For this review, take the finished solid that the model builds, in its own axes (mm). Face numbers are marked on the shaded views. Coordinates: 2 decimals unless noted, no trailing zeros. Write each loop counter-clockwise with the first axis right and the second up, starting at its lowest first coordinate (ties: lowest second). Pieces come first, ordered by that corner, then holes.
```python
from build123d import *

# Parameters (mm, degrees)
CROQUIS1_W              = 44
CROQUIS1_H              = 35.7
CROQUIS1_R              = 14
SALIENTE_EXTRUIR1_DEPTH = 5.4


with BuildPart() as part:
    # Croquis1 → Saliente-Extruir1 (new body)
    with BuildSketch(Plane.XY):
        Rectangle(CROQUIS1_W, CROQUIS1_H)
        with Locations(Location((0, 0, 0), (0, 0, 180))):
            Circle(CROQUIS1_R, mode=Mode.SUBTRACT)
    extrude(amount=SALIENTE_EXTRUIR1_DEPTH)


solid = part.part
```
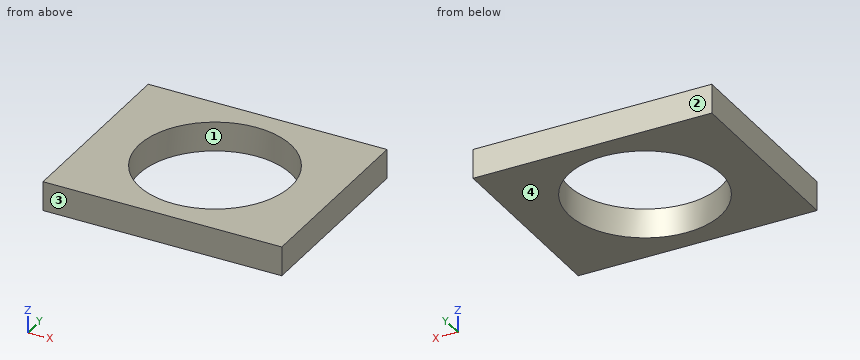
1) Clearance check with flat-ended pins moving along their axes: P1, Ø6, axis at x = 11, y = 6, coming from the -Z side; P2, Ø8, axis at x = 3.5, y = -5, coming from the -Z side. State where each tip first meets the part, or that it passes through.
2) The part is to be moulded in two halves that separate along Y. For the marked faces 1, 2, 3 and 4, say which applies: pulls with the +Y half, pulls with the -Y half, needs draft (parallel to the pull), parting line crosses it, or undercut.
3) Consider section B-B (y = 0). Give the boundary of the cut face in (x, z).
4) For L1, parallel to Y at x = 0, z = 1.8; L2, parallel to Y at x = -3, z = 4.8; L3, parallel to X at y = 3, z = 2.7, list the stretches that pass through material, from the lowest coordinate up.
5) Consider section A-A (x = 0). Give the boundary of the cut face in (y, z), then the cut area to 3 significant figures.
6) Consider section C-C (z = 3.35). Give the boundary of the cut face in (x, y).
Results:
1. P1: stops at z = 0
1. P2: passes through
2. face 1: undercut
2. face 2: pulls with the +Y half
2. face 3: pulls with the -Y half
2. face 4: needs draft
3. outline: (-22, 0) - (-14, 0) - (-14, 5.4) - (-22, 5.4) - close; (14, 0) - (22, 0) - (22, 5.4) - (14, 5.4) - close
4. L1: y = -17.85 to -14, 14 to 17.85
4. L2: y = -17.85 to -13.67, 13.67 to 17.85
4. L3: x = -22 to -13.67, 13.67 to 22
5. outline: (-17.85, 0) - (-14, 0) - (-14, 5.4) - (-17.85, 5.4) - close; (14, 0) - (17.85, 0) - (17.85, 5.4) - (14, 5.4) - close
5. area: 41.6 mm2
6. outline: (-22, -17.85) - (22, -17.85) - (22, 17.85) - (-22, 17.85) - close; hole circle Ø28 at (0, 0)
